Read the model definition and answer for the solid it produces. Units are mm, in the model's axes. A direction names the side the tool comes from. Give positions to 0.01 mm unless a question says otherwise; leave off trailing zeros. Loops run counter-clockwise (first coordinate to the right, second up) from the corner with the lowest first, then second, coordinate; pieces in that order, holes last. Notation, with made-up numbers: (81, 41) -> (91, 41) arc R15 ccw to (91, 62) -> close; hole circle Ø3 at (-31, -14.5). An arc over 180 degrees is marked (long way). One line per item, written item: value. Start each with the question number.
from build123d import *

# Parameters (mm, degrees)
SKETCH1_R           = 101.6
SKETCH1_R_2         = 2.1525
SKETCH1_R_3         = 2.1524976
BOSS_EXTRUDE1_DEPTH = 6.35
FILLET1_R           = 7.5


with BuildPart() as part:
    # Sketch1 → Boss-Extrude1 (new body)
    with BuildSketch(Plane.XY):
        with BuildLine():
            Line((115.326459663, 17), (143.1000104, 17))
            ThreePointArc((143.1000104, 17), (148.403311259, 14.803300859), (150.6000104, 9.5))
            Line((150.6000104, 9.5), (150.6000104, -9.5))
            ThreePointArc((150.6000104, -9.5), (148.403311259, -14.803300859), (143.1000104, -17))
            Line((143.1000104, -17), (115.326459663, -17))
            ThreePointArc((115.326459663, -17), (0, -116.572691049), (-115.326459663, -17))
            Line((-115.326459663, -17), (-143.1000104, -17))
            ThreePointArc((-143.1000104, -17), (-148.403311259, -14.803300859), (-150.6000104, -9.5))
            Line((-150.6000104, -9.5), (-150.6000104, 9.5))
            ThreePointArc((-150.6000104, 9.5), (-148.403311259, 14.803300859), (-143.1000104, 17))
            Line((-143.1000104, 17), (-115.326459663, 17))
            ThreePointArc((-115.326459663, 17), (0, 116.572691049), (115.326459663, 17))
        make_face()
        Circle(SKETCH1_R, mode=Mode.SUBTRACT)
        with Locations((133.6000104, 9.5)):
            Circle(SKETCH1_R_2, mode=Mode.SUBTRACT)
        with Locations((133.6000104, -9.5)):
            Circle(SKETCH1_R_2, mode=Mode.SUBTRACT)
        with Locations((143.1000104, 0)):
            Circle(SKETCH1_R_2, mode=Mode.SUBTRACT)
        with Locations((124.1000104, 0)):
            Circle(SKETCH1_R_2, mode=Mode.SUBTRACT)
        with Locations(Location((-143.1000104, 0, 0), (0, 0, 180))):
            Circle(SKETCH1_R_2, mode=Mode.SUBTRACT)
        with Locations(Location((-133.6000104, -9.5, 0), (0, 0, 180))):
            Circle(SKETCH1_R_2, mode=Mode.SUBTRACT)
        with Locations(Location((-124.1000104, 0, 0), (0, 0, 180))):
            Circle(SKETCH1_R_2, mode=Mode.SUBTRACT)
        with Locations(Location((-133.6000104, 9.5, 0), (0, 0, 180))):
            Circle(SKETCH1_R_2, mode=Mode.SUBTRACT)
        with Locations((0, 109.22)):
            Circle(SKETCH1_R_3, mode=Mode.SUBTRACT)
        with Locations((22.708114871, 106.833280952)):
            Circle(SKETCH1_R_3, mode=Mode.SUBTRACT)
        with Locations((44.423776157, 99.777434884)):
            Circle(SKETCH1_R_3, mode=Mode.SUBTRACT)
        with Locations((64.197905255, 88.360836126)):
            Circle(SKETCH1_R_3, mode=Mode.SUBTRACT)
        with Locations((81.166277839, 73.082444827)):
            Circle(SKETCH1_R_3, mode=Mode.SUBTRACT)
        with Locations((94.587294601, 54.61)):
            Circle(SKETCH1_R_3, mode=Mode.SUBTRACT)
        with Locations((103.87439271, 33.750836126)):
            Circle(SKETCH1_R_3, mode=Mode.SUBTRACT)
        with Locations((108.621681412, 11.416598758)):
            Circle(SKETCH1_R_3, mode=Mode.SUBTRACT)
        with Locations((108.621681412, -11.416598758)):
            Circle(SKETCH1_R_3, mode=Mode.SUBTRACT)
        with Locations((103.87439271, -33.750836126)):
            Circle(SKETCH1_R_3, mode=Mode.SUBTRACT)
        with Locations((94.587294601, -54.61)):
            Circle(SKETCH1_R_3, mode=Mode.SUBTRACT)
        with Locations((81.166277839, -73.082444827)):
            Circle(SKETCH1_R_3, mode=Mode.SUBTRACT)
        with Locations((64.197905255, -88.360836126)):
            Circle(SKETCH1_R_3, mode=Mode.SUBTRACT)
        with Locations((44.423776157, -99.777434884)):
            Circle(SKETCH1_R_3, mode=Mode.SUBTRACT)
        with Locations((22.708114871, -106.833280952)):
            Circle(SKETCH1_R_3, mode=Mode.SUBTRACT)
        with Locations((0, -109.22)):
            Circle(SKETCH1_R_3, mode=Mode.SUBTRACT)
        with Locations((-22.708114871, -106.833280952)):
            Circle(SKETCH1_R_3, mode=Mode.SUBTRACT)
        with Locations((-44.423776157, -99.777434884)):
            Circle(SKETCH1_R_3, mode=Mode.SUBTRACT)
        with Locations((-64.197905255, -88.360836126)):
            Circle(SKETCH1_R_3, mode=Mode.SUBTRACT)
        with Locations((-81.166277839, -73.082444827)):
            Circle(SKETCH1_R_3, mode=Mode.SUBTRACT)
        with Locations((-94.587294601, -54.61)):
            Circle(SKETCH1_R_3, mode=Mode.SUBTRACT)
        with Locations((-103.87439271, -33.750836126)):
            Circle(SKETCH1_R_3, mode=Mode.SUBTRACT)
        with Locations((-108.621681412, -11.416598758)):
            Circle(SKETCH1_R_3, mode=Mode.SUBTRACT)
        with Locations((-108.621681412, 11.416598758)):
            Circle(SKETCH1_R_3, mode=Mode.SUBTRACT)
        with Locations((-103.87439271, 33.750836126)):
            Circle(SKETCH1_R_3, mode=Mode.SUBTRACT)
        with Locations((-94.587294601, 54.61)):
            Circle(SKETCH1_R_3, mode=Mode.SUBTRACT)
        with Locations((-81.166277839, 73.082444827)):
            Circle(SKETCH1_R_3, mode=Mode.SUBTRACT)
        with Locations((-64.197905255, 88.360836126)):
            Circle(SKETCH1_R_3, mode=Mode.SUBTRACT)
        with Locations((-44.423776157, 99.777434884)):
            Circle(SKETCH1_R_3, mode=Mode.SUBTRACT)
        with Locations((-22.708114871, 106.833280952)):
            Circle(SKETCH1_R_3, mode=Mode.SUBTRACT)
    extrude(amount=BOSS_EXTRUDE1_DEPTH)

    # Fillet1
    fillet1_edges = [part.edges().sort_by_distance(p)[0] for p in [
        (115.326459663, 17, 3.175),
        (115.326459663, -17, 3.175),
        (-115.326459663, -17, 3.175),
        (-115.326459663, 17, 3.175),
    ]]
    fillet(fillet1_edges, radius=FILLET1_R)


solid = part.part
Item 1: Flat-ended cylindrical pins translate along their axes: pin 1 (1 mm diameter, centred on x = 49, z = 4.5, fed in from -Y); pin 2 (2 mm diameter, centred on x = 108, z = 3, fed in from -Y); pin 3 (3 mm diameter, centred on x = -130, z = 3, fed in from -Y). Find the tip coordinate at first contact, or state that the pin passes through.
Item 2: For faces 1 (the flat face through (132, 17, 3)), 2 (the flat face through (-133, 17, 3)), 3 (the flat face through (-55, -86, 0)), 4 (the flat face through (-132, -17, 3)), 5 (the flat face through (-55, -86, 6.35)), determine the directions among +Z, -Z, +X, -X, +Y, -Y from which every point of the face is accessible in a straight line to the end or side of a thin tool.
Item 3: Section A-A, the plane y = -48 is taken. Determine the outline of the cut face in (x, z).
Item 4: Determine the mould class of faces 6 (the cylindrical face through (-148.461, 14.745, 3.131)), 7 (the flat face through (150.6, 0, 3)), 8 (the cylindrical face through (-22.025, -99.184, 3.131)), 9 (the cylindrical face through (-2.24, 116.55, 3.13)) for opening direction X: pulls with the +X half, pulls with the -X half, needs draft (parallel to the pull), parting line crosses it, or undercut.
Item 5: Section B-B, the plane z = 1.25 is taken. State how many separate pieces and enclosed holes the cut face has, plus the area to 3 significant figures.
Item 6: Consider L1, parallel to X at y = -1, z = 1.75; L2, parallel to Y at x = -80.5, z = 2.75; L3, parallel to X at y = -10.5, z = 2.25. Determine where each line is inside the solid, lowest interval first. Write a range as [from, to].
Computed values:
1. pin 1: y = -106
1. pin 2: y = -46.26
1. pin 3: y = -17
2. face 1: +Z, -Z, +X, +Y
2. face 2: +Z, -Z, -X, +Y
2. face 3: -Z, +X, -X, +Y, -Y
2. face 4: +Z, -Z, -X, -Y
2. face 5: +Z, +X, -X, +Y, -Y
3. outline: (-106.23, 0) -> (-89.55, 0) -> (-89.55, 6.35) -> (-106.23, 6.35) -> close; (89.55, 0) -> (106.23, 0) -> (106.23, 6.35) -> (89.55, 6.35) -> close
4. face 6: pulls with the -X half
4. face 7: pulls with the +X half
4. face 8: undercut
4. face 9: parting line crosses it
5. separate pieces: 1
5. enclosed holes: 39
5. area: 12,000 mm²
6. L1: [-150.6, -145.01], [-141.19, -126.01], [-122.19, -101.6], [101.6, 122.19], [126.01, 141.19], [145.01, 150.6]
6. L2: [-84.31, -75.13], [-71.04, -61.99], [61.99, 71.04], [75.13, 84.31]
6. L3: [-150.53, -135.51], [-131.69, -110.57], [-106.67, -101.06], [101.06, 106.67], [110.57, 131.69], [135.51, 150.53]
